Build history of the part. All positions in model axes, mm. A direction names the side the tool comes from. Give positions to 0.01 mm unless a question says otherwise; leave off trailing zeros. Write each loop counter-clockwise with the first axis right and the second up, starting at its lowest first coordinate (ties: lowest second). Pieces come first, ordered by that corner, then holes. Notation, with made-up numbers: (-38.75, -8.75) -> (-24.75, -8.75) arc R10 cw to (-24.75, -2.75) -> close; hole circle Ø10 at (-23.5, 49.5). An arc over 180 degrees is marked (long way). Put each result on its own line as item: value. Start each with the question number.
Item 1: Flat gauge pins, fed straight in: pin 1 Ø1.3 at (x, y) = (0, 11.5) entering from -Z; pin 2 Ø3 at (x, z) = (-19, -34) entering from +Y; pin 3 Ø2 at (x, y) = (0, 11.5) entering from +Z. Where does each tip first touch, or does it go through?
Item 2: Slice it at C-C, the plane z = -0.5. List the corners of the cut face in (x, y), plus the area to 3 significant figures.
Item 3: Slice it at A-A, the plane x = 28. List the corners of the cut face in (y, z), plus the area to 3 significant figures.
Item 4: Two-plate mould, pull along Z, no slides. Class faces 4 (the flat face through (35, 4, -36)), 5 (the flat face through (0, 10, 40.5)), 6 (the flat face through (0, 7, 50.5)): pulls with the +Z half, pulls with the -Z half, needs draft (parallel to the pull), parting line crosses it, or undercut.
Item 5: Drill centre lines: line 1 along Y through (x, z) = (0, 49); line 2 along X through (y, z) = (2.4, 21.5); line 3 along X through (y, z) = (1.25, 12). Where is each one in solid material? Low to high.
Item 6: Slice it at D-D, the plane y = 7.75. List the corners of the cut face in (x, z).
Item 7: Slice it at B-B, the plane z = 21.5. List the corners of the cut face in (x, y), plus the area to 3 significant figures.
Item 8: Tool access for faces 1 (the flat face through (27, 3, 15)), 2 (the flat face through (-19, 3, 0)), 3 (the cylindrical face through (0.421, 12.516, -47.369)): list every direction of +Z, -Z, +X, -X, +Y, -Y with a clear straight run to the whole face (end or side of a thin tool).
```python
from build123d import *

# Parameters (mm, degrees)
SKETCH_1_W           = 70
SKETCH_1_H           = 101
EXTRUDE_1_DEPTH      = 15
SKETCH_3_W           = 70
SKETCH_3_H           = 81
CUT_EXTRUDE_2_DEPTH  = 10
F_1_0MM_1_AT_2_COUNT = 2
F_1_0MM_1_AT_2_PITCH = 8
SKETCH_7_W           = 16
SKETCH_7_H           = 30
CUT_EXTRUDE_3_DEPTH  = 63.251506006
F_1_0MM_3_D          = 2.2
SKETCH_11_R          = 5
CUT_EXTRUDE_4_DEPTH  = 64.247529596
F_1_0MM_2_D          = 2.2


with BuildPart() as part:
    # 草圖1 → 填料-伸長1 (new body)
    with BuildSketch(Plane(origin=(0, 0, 0), x_dir=(1, 0, 0), z_dir=(0, 1, 0))):
        Rectangle(SKETCH_1_W, SKETCH_1_H)
    extrude(amount=EXTRUDE_1_DEPTH)

    # 草圖3 → 除料-伸長2 (cut)
    with BuildSketch(Plane(origin=(0, 15, 0), x_dir=(1, 0, 0), z_dir=(0, 1, 0))):
        Rectangle(SKETCH_3_W, SKETCH_3_H)
    extrude(amount=-CUT_EXTRUDE_2_DEPTH, mode=Mode.SUBTRACT)

    # 草圖6 → Ø1.0mm 定位孔1 (revolve, cut)
    with BuildSketch(Plane(origin=(0, 3.5, -50.5), x_dir=(0, 1, 0), z_dir=(1, 0, 0))):
        Polygon((0, 0), (0, 7.010946681), (1.1, 6.35), (1.1, 0), align=None)
    f_1_0mm_1 = revolve(axis=Axis((0, 3.5, -56.85), (0, 0, 1)), mode=Mode.SUBTRACT)

    # Ø1.0mm 定位孔1 at 2: Ø1.0mm 定位孔1 ×2
    with Locations(*[(0, i * F_1_0MM_1_AT_2_PITCH, 0) for i in range(1, F_1_0MM_1_AT_2_COUNT)]):
        add(f_1_0mm_1, mode=Mode.SUBTRACT)

    # 鏡射1: Ø1.0mm 定位孔1 across plane
    add(f_1_0mm_1.mirror(Plane.XY), mode=Mode.SUBTRACT)

    # 鏡射1 copy 1 sketch → 鏡射1 copy 1 (revolve, cut)
    with BuildSketch(Plane(origin=(0, 11.5, 50.5), x_dir=(0, 1, 0), z_dir=(1, 0, 0))):
        Polygon((0, 0), (0, -7.010946681), (1.1, -6.35), (1.1, 0), align=None)
    revolve(axis=Axis((0, 11.5, 56.85), (0, 0, 1)), mode=Mode.SUBTRACT)

    # 草圖7 → 除料-伸長3 (cut, through all)
    with BuildSketch(Plane(origin=(0, 5, 0), x_dir=(1, 0, 0), z_dir=(0, 1, 0))):
        with Locations((27, 0)):
            Rectangle(SKETCH_7_W, SKETCH_7_H)
    cut_extrude_3 = extrude(amount=-CUT_EXTRUDE_3_DEPTH, mode=Mode.SUBTRACT)

    # 鏡射2: 除料-伸長3 across plane
    add(cut_extrude_3.mirror(Plane(origin=(0, 0, 0), x_dir=(0, 0, 1), z_dir=(1, 0, 0))), mode=Mode.SUBTRACT)

    # Ø1.0mm 定位孔3 (through all)
    with Locations(Plane(origin=(0, 0, 0), x_dir=(-1, 0, 0), z_dir=(0, -1, 0))):
        with Locations((-12.5, -12), (12.5, -12), (-12.5, 12), (12.5, 12)):
            Hole(F_1_0MM_3_D / 2)

    # 草圖11 → 除料-伸長4 (cut, through all)
    with BuildSketch(Plane.XZ):
        with Locations(Location((-12.5, -4.5, 0), (0, 0, 270))):
            Circle(SKETCH_11_R)
    extrude(amount=-CUT_EXTRUDE_4_DEPTH, mode=Mode.SUBTRACT)

    # Ø1.0mm 定位孔2 (through all)
    with Locations(Plane(origin=(0, 5, 0), x_dir=(1, 0, 0), z_dir=(0, 1, 0))):
        with Locations((-19, 34), (-19, 21.5), (19, 21.5), (19, 34)):
            f_1_0mm_2 = Hole(F_1_0MM_2_D / 2)

    # 鏡射3: Ø1.0mm 定位孔2 across plane
    add(f_1_0mm_2.mirror(Plane.XY), mode=Mode.SUBTRACT)


solid = part.part
```
Values follow:
1. pin 1: z = -43.88
1. pin 2: y = 5
1. pin 3: z = 44.09
2. outline: (-19, 0) -> (-15.5, 0) -> (-15.5, 5) -> (-19, 5) -> close; (-9.5, 0) -> (19, 0) -> (19, 5) -> (-9.5, 5) -> close
2. area: 160 mm2
3. outline: (0, -50.5) -> (15, -50.5) -> (15, -40.5) -> (5, -40.5) -> (5, -15) -> (0, -15) -> close; (0, 15) -> (5, 15) -> (5, 40.5) -> (15, 40.5) -> (15, 50.5) -> (0, 50.5) -> close
3. area: 555 mm2
4. face 4: needs draft
4. face 5: undercut
4. face 6: pulls with the +Z half
5. line 1: 0 to 2.4, 4.6 to 10.4, 12.6 to 15
5. line 2: -35 to -20.1, -17.9 to 17.9, 20.1 to 35
5. line 3: -19 to -13.6, -11.4 to 11.4, 13.6 to 19
6. outline: (-35, -50.5) -> (35, -50.5) -> (35, -40.5) -> (-35, -40.5) -> close; (-35, 40.5) -> (35, 40.5) -> (35, 50.5) -> (-35, 50.5) -> close
7. outline: (-35, 0) -> (-20.1, 0) -> (-20.1, 5) -> (-35, 5) -> close; (-17.9, 0) -> (17.9, 0) -> (17.9, 5) -> (-17.9, 5) -> close; (20.1, 0) -> (35, 0) -> (35, 5) -> (20.1, 5) -> close
7. area: 328 mm2
8. face 1: +X, +Y, -Y
8. face 2: -X, +Y, -Y
8. face 3: -Z
